from build123d import *

# Parameters (mm, degrees)
F0_W     = 129.9482808348
F0_H     = 127
F1_DEPTH = 25.4
F2_W     = 25.4
F2_H     = 127
F3_DEPTH = 25.4
F4_DEPTH = 76.2
F5_W     = 104.5482808348
F5_H     = 21.0354196131
F6_DEPTH = 101.6
F7_W     = 25.4
F7_H     = 25.4
F8_DEPTH = 25.4


with BuildPart() as f1:
    # F0 (on Top) → F1 (new body)
    with BuildSketch(Plane.XY):
        with Locations((7.7071934938, 2.8795562685)):
            Rectangle(F0_W, F0_H)
    extrude(amount=F1_DEPTH)

    # F2 (on face) → F3 (join)
    with BuildSketch(Plane.XY.offset(25.4)):
        with Locations((-44.5669469236, 2.8795562685)):
            Rectangle(F2_W, F2_H)
    extrude(amount=F3_DEPTH)

    # F4 (add): a face of the model
    f4_faces = [f1.faces().sort_by_distance(p)[0] for p in [
        (-44.5669469236, 2.8795562685, 50.8),
    ]]
    extrude(f4_faces, amount=F4_DEPTH)

    # F5 (on face) → F6 (join)
    with BuildSketch(Plane.XY.offset(25.4)):
        with Locations((20.4071934938, 55.8618464619)):
            Rectangle(F5_W, F5_H)
    extrude(amount=F6_DEPTH)

    # F7 (on face) → F8 (cut)
    with BuildSketch(Plane.XY.offset(25.4)):
        with Locations((59.9813339112, -47.9204437315)):
            Rectangle(F7_W, F7_H)
    extrude(amount=-F8_DEPTH, mode=Mode.SUBTRACT)


solid = f1.part
Build history of the part. All positions in model axes, mm. A direction names the side the tool comes from. Round coordinates to 2 decimals unless told otherwise and drop trailing zeros. Loops run counter-clockwise (first coordinate to the right, second up) from the corner with the lowest first, then second, coordinate; pieces in that order, holes last. Notation, with made-up numbers: (75.25, -21) -> (130.25, -21) arc R26 ccw to (130.25, 4) -> close; hole circle Ø10 at (72, 1.5). An arc over 180 degrees is marked (long way). One line per item, written item: value. Start each with the question number.
Q1. Cut at B-B on x = 55. List the corners of the cut face in (y, z).
Q2. Cut at A-A on z = 23. List the corners of the cut face in (x, y), plus the area to 3 significant figures.
Q3. Drop flat-ended pins along their axis: pin 1 Ø6 at (x, y) = (-18.5, -1.5) entering from +Z; pin 2 Ø1 at (x, z) = (-31, 61.5) entering from -Y; pin 3 Ø12.5 at (y, z) = (-45, 11) entering from +X. Give the stop position or say it passes through.
Q4. Two-plate mould, pull along X, no slides. Class faces 1 (the face through (-41, -60.62, 34)), 2 (the face through (-57.267, 2, 63)), 3 (the face through (47.281, -48, 13)): released by +X, released by -X, zero draft, split by the parting line, or undercut.
Q5. Probe line 1 along Y through (x, z) = (-6, 84); line 2 along X through (y, z) = (42, 46); line 3 along Z through (x, y) = (45, 31.5). List the from-to ranges inside material, lowest first.
Q6. 3-axis set-ups, long thin cutter, end or side, ignore diameter. For faces 4 (the face through (60, -35.22, 13)), 5 (the face through (7, 66.38, 63)), 6 (the face through (-31.867, -8, 75)): which of +Z, -Z, +X, -X, +Y, -Y reach the whole face in a straight line?
Computed:
1. outline: (-35.22, 0) -> (66.38, 0) -> (66.38, 127) -> (45.34, 127) -> (45.34, 25.4) -> (-35.22, 25.4) -> close
2. outline: (-57.27, -60.62) -> (47.28, -60.62) -> (47.28, -35.22) -> (72.68, -35.22) -> (72.68, 66.38) -> (-57.27, 66.38) -> close
2. area: 15,900 mm²
3. pin 1: z = 25.4
3. pin 2: y = 45.34
3. pin 3: x = 47.28
4. face 1: zero draft
4. face 2: released by -X
4. face 3: released by +X
5. line 1: 45.34 to 66.38
5. line 2: -57.27 to -31.87
5. line 3: 0 to 25.4
6. face 4: +Z, -Z, +X, -Y
6. face 5: +Z, -Z, +X, -X, +Y
6. face 6: +Z, +X, -Y
